```python
from build123d import *

# Parameters (mm, degrees)
SKETCH_1_W                   = 196
SKETCH_1_H                   = 196
EXTRUDE_1_DEPTH              = 17
HOLE_WIZARD_1_D              = 8.376
HOLE_WIZARD_M241_D           = 26
HOLE_WIZARD_M241_CBORE_D     = 32
HOLE_WIZARD_M241_CBORE_DEPTH = 6.3
CHAMFER_1_SIZE               = 0.812


with BuildPart() as part:
    # Эскиз1 → Бобышка-Вытянуть1 (new body)
    with BuildSketch(Plane.XY.offset(17)):
        Rectangle(SKETCH_1_W, SKETCH_1_H)
    extrude(amount=-EXTRUDE_1_DEPTH)

    # Отверстие1 (through all)
    with Locations(Plane.XY.offset(17)):
        with Locations((-50, 77), (-50, -77), (50, 77), (50, -77)):
            Hole(HOLE_WIZARD_1_D / 2)

    # Цековка для  болта с шестигранной головкой M241 (through all)
    with Locations(Plane.XY.offset(17)):
        with Locations((76, -77), (-76, -77), (76, 77), (-76, 77)):
            CounterBoreHole(HOLE_WIZARD_M241_D / 2, HOLE_WIZARD_M241_CBORE_D / 2, HOLE_WIZARD_M241_CBORE_DEPTH)

    # Фаска1
    chamfer_1_edges = [part.edges().sort_by_distance(p)[0] for p in [
        (54.188, -77, 17),
        (54.188, 77, 17),
        (-45.812, -77, 17),
        (-45.812, 77, 17),
    ]]
    chamfer(chamfer_1_edges, length=CHAMFER_1_SIZE)


solid = part.part
```
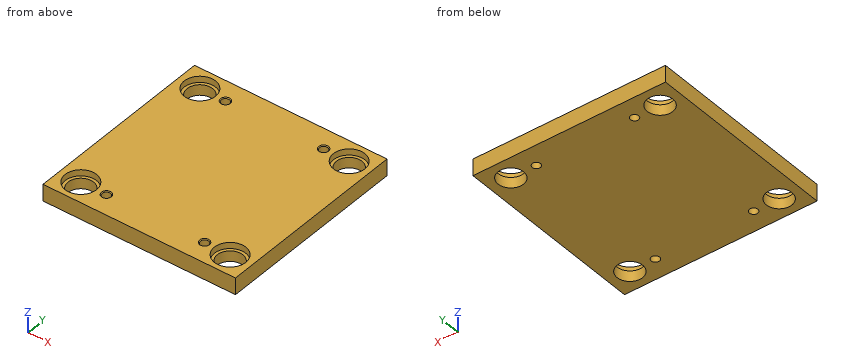
Here's how the part is built. I have some questions about the finished solid (model axes, mm). Give positions to 0.01 mm unless a question says otherwise; leave off trailing zeros. Order: outer loops, then holes, each group sorted by start corner. A loop starts at its lowest first (then second) coordinate and runs counter-clockwise, first axis right, second up. Notation, with made-up numbers: (61, 24) - (66, 24) arc R18 cw to (66, 55) - close; hole circle Ø4 at (77, 29). An arc over 180 degrees is marked (long way). Answer as a JSON object with one key per item and string values. Group by question number.
Item 1: If we section it at D-D on y = -84.5: Please give me the cut outline in (x, z).
Item 2: If we section it at A-A on y = 77: Give the number of separate pieces and of enclosed holes in the cut face, and give its area (3 significant figures).
Item 3: If we section it at C-C on x = -76: Please give me the cut outline in (y, z).
Item 4: Please list where these lines run through material, in increasing order: probe 1 along Y at (x, z) = (76, 8); probe 2 along Y at (x, z) = (75, 16); probe 3 along X at (y, z) = (-66, 3).
Item 5: For P1, Ø15.5, axis at x = 76, y = -77, coming from the +Z side; P2, Ø9.5, axis at x = -50, y = -77, coming from the -Z side, each with a flat end and sliding along its axis, tell me the tip position at first contact or that it passes through.
Result set:
{
 "1": {"outline": "(-98, 0) - (-86.62, 0) - (-86.62, 10.7) - (-90.13, 10.7) - (-90.13, 17) - (-98, 17) - close; (-65.38, 0) - (65.38, 0) - (65.38, 10.7) - (61.87, 10.7) - (61.87, 17) - (-61.87, 17) - (-61.87, 10.7) - (-65.38, 10.7) - close; (86.62, 0) - (98, 0) - (98, 17) - (90.13, 17) - (90.13, 10.7) - (86.62, 10.7) - close"},
 "2": {"separate pieces": "5", "enclosed holes": "0", "area": "2,090 mm²"},
 "3": {"outline": "(-98, 0) - (-90, 0) - (-90, 10.7) - (-93, 10.7) - (-93, 17) - (-98, 17) - close; (-64, 0) - (64, 0) - (64, 10.7) - (61, 10.7) - (61, 17) - (-61, 17) - (-61, 10.7) - (-64, 10.7) - close; (90, 0) - (98, 0) - (98, 17) - (93, 17) - (93, 10.7) - (90, 10.7) - close"},
 "4": {"probe 1": "-98 to -90, -64 to 64, 90 to 98", "probe 2": "-98 to -92.97, -61.03 to 61.03, 92.97 to 98", "probe 3": "-98 to -82.93, -69.07 to 69.07, 82.93 to 98"},
 "5": {"P1": "through", "P2": "z = 0"}
}
